Build history of the part. All positions in model axes, mm. A direction names the side the tool comes from. Give positions to 0.01 mm unless a question says otherwise; leave off trailing zeros. Order: outer loops, then holes, each group sorted by start corner. A loop starts at its lowest first (then second) coordinate and runs counter-clockwise, first axis right, second up. Notation, with made-up numbers: M 28.25,-28.75 L 32.25,-28.75 A27 cw 32.25,10.25 Z; hole C -28.75,50.5 d1. An arc over 180 degrees is marked long. Use CSV: the item, a comma, the result in double quotes. Start each with the question number.
Item 1: Band-saw the part on C-C on x = 69. Write the cut outline in (y, z), plus the area to 3 significant figures.
Item 2: Band-saw the part on B-B on x = 53. Write the cut outline in (y, z), plus the area to 3 significant figures.
Item 3: Band-saw the part on A-A on z = 12.25. Write the cut outline in (x, y).
Item 4: Wall check: line 1 along X through (y, z) = (43.2, 8); line 2 along Y through (x, z) = (17.5, 14); line 3 along Z through (x, y) = (48, 127). Give the ranges that are in metal, low to high.
Item 5: Pin check, flat tips, straight feed: P1, Ø2, axis at x = 54, y = 76.5, coming from the +Z side; P2, Ø3, axis at y = 90, z = 5.5, coming from the +X side. Stop position of each tip, or through.
Item 6: Two-plate mould, pull along Z, no slides. Class faces 1 (the flat face through (37, 96, 3)), 2 (the cylindrical face through (24.537, 146.479, 8.202)), 3 (the flat face through (76, 95, 2)): pulls with the +Z half, pulls with the -Z half, needs draft (parallel to the pull), parting line crosses it, or undercut.
Item 7: Band-saw the part on D-D on y = 66. Write the cut outline in (x, z), plus the area to 3 significant figures.
Item 8: Which spindle directions (+Z, -Z, +X, -X, +Y, -Y) get a long thin tool onto all of the face, cutting with end or side? Do faces 4 (the flat face through (0, 95, 2)), 5 (the flat face through (37, 45, 9)). Say none if no direction does.
from build123d import *

# Parameters (mm, degrees)
SKETCH_1_W          = 76
SKETCH_1_H          = 190
SKETCH_1_R          = 1.55
EXTRUDE_1_DEPTH     = 3
SKETCH_2_W          = 76
SKETCH_2_H          = 3
EXTRUDE_2_DEPTH     = 12
SKETCH_3_R          = 1.55
CUT_EXTRUDE_1_DEPTH = 168.047897323
SKETCH_4_W          = 76
SKETCH_4_H          = 42
CUT_EXTRUDE_2_DEPTH = 10


with BuildPart() as part:
    # 草图1 → 凸台-拉伸1 (new body)
    with BuildSketch(Plane.XY):
        with Locations((38, 95)):
            Rectangle(SKETCH_1_W, SKETCH_1_H)
        with Locations((63, 10)):
            Circle(SKETCH_1_R, mode=Mode.SUBTRACT)
        with Locations((13, 10)):
            Circle(SKETCH_1_R, mode=Mode.SUBTRACT)
        with Locations((63, 180)):
            Circle(SKETCH_1_R, mode=Mode.SUBTRACT)
        with Locations((13, 180)):
            Circle(SKETCH_1_R, mode=Mode.SUBTRACT)
    extrude(amount=EXTRUDE_1_DEPTH)

    # 草图2 → 凸台-拉伸2 (add)
    with BuildSketch(Plane.XY.offset(3)):
        with Locations((38, 43.5)):
            Rectangle(SKETCH_2_W, SKETCH_2_H)
        with Locations((38, 146.5)):
            Rectangle(SKETCH_2_W, SKETCH_2_H)
    extrude(amount=EXTRUDE_2_DEPTH)

    # 草图3 → 切除-拉伸1 (cut, through all)
    with BuildSketch(Plane.XZ.offset(-42)):
        with Locations(Location((23, 8, 0), (0, 0, 270))):
            Circle(SKETCH_3_R)
        with Locations(Location((53, 8, 0), (0, 0, 270))):
            Circle(SKETCH_3_R)
    extrude(amount=-CUT_EXTRUDE_1_DEPTH, mode=Mode.SUBTRACT)

    # 草图4 → 切除-拉伸2 (cut)
    with BuildSketch(Plane.XY.offset(3)):
        with Locations((38, 21)):
            Rectangle(SKETCH_4_W, SKETCH_4_H)
        with Locations((38, 169)):
            Rectangle(SKETCH_4_W, SKETCH_4_H)
    extrude(amount=-CUT_EXTRUDE_2_DEPTH, mode=Mode.SUBTRACT)


solid = part.part
Model answer:
1,outline,"M 42,0 L 148,0 L 148,15 L 145,15 L 145,3 L 45,3 L 45,15 L 42,15 Z"
1,area,"390 mm^2"
2,outline,"M 42,0 L 148,0 L 148,6.45 L 145,6.45 L 145,3 L 45,3 L 45,6.45 L 42,6.45 Z; M 42,9.55 L 45,9.55 L 45,15 L 42,15 Z; M 145,9.55 L 148,9.55 L 148,15 L 145,15 Z"
2,area,"371 mm^2"
3,outline,"M 0,42 L 76,42 L 76,45 L 0,45 Z; M 0,145 L 76,145 L 76,148 L 0,148 Z"
4,line 1,"x = 0 to 21.45, 24.55 to 51.45, 54.55 to 76"
4,line 2,"y = 42 to 45, 145 to 148"
4,line 3,"z = 0 to 3"
5,P1,"stops at z = 3"
5,P2,"passes through"
6,face 1,"pulls with the +Z half"
6,face 2,"undercut"
6,face 3,"needs draft"
7,outline,"M 0,0 L 76,0 L 76,3 L 0,3 Z"
7,area,"228 mm^2"
8,face 4,"+Z, -Z, -X, +Y, -Y"
8,face 5,"+Z, +X, -X"
